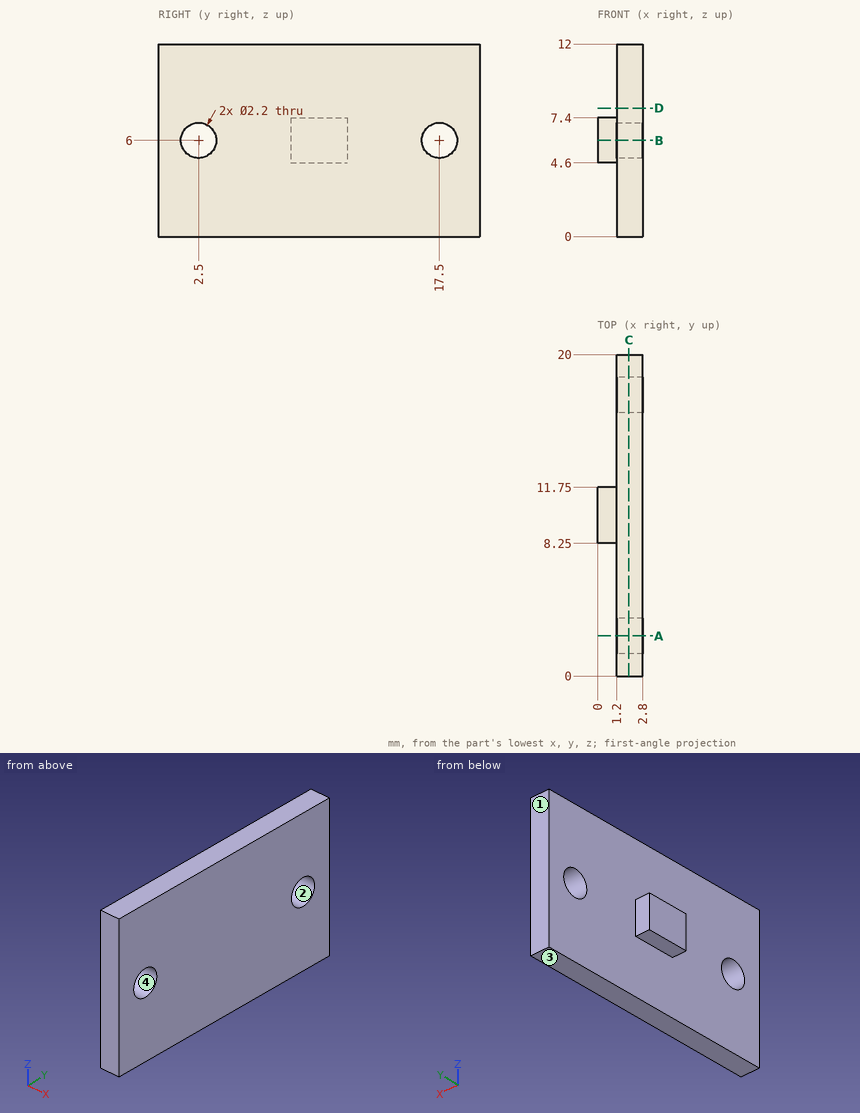
Could you check a few things on this drawing? It's one solid part, dimensions in mm from its lowest x, y, z. Coordinates: 2 decimals unless noted, no trailing zeros. Order: outer loops, then holes, each group sorted by start corner. A loop starts at its lowest first (then second) coordinate and runs counter-clockwise, first axis right, second up. Notation, with made-up numbers: M -30.5,35 L 2.5,35 A27 cw 2.5,60 Z; hole C 37.25,-19.5 d9. An arc over 180 degrees is marked long. Use one line per item in the form item = value. Start each with the question number.
1. Suppose I cut it at A-A on y = 2.5. Write out the boundary of the cut face in (x, z).
2. Suppose I cut it at C-C on x = 1.95. Write out the boundary of the cut face in (y, z), then the cut area to 3 significant figures.
3. Suppose I cut it at D-D on z = 8. Write out the boundary of the cut face in (x, y).
4. Please list where these lines run through material, in increasing order: line 1 (Y direction, x = 2.45, z = 6); line 2 (X direction, y = 6.75, z = 1.75); line 3 (Z direction, x = 2.2, y = 3.25).
5. We'd pull the mould along Z, two halves only. Please class the marked faces 1, 2, 3 and 4: +Z half, -Z half, draft (parallel to the pull), parting line (faces both ways), or undercut.
6. For pin 1 (1 mm diameter, centred on y = 5.5, z = 9.5, fed in from -X); pin 2 (1.3 mm diameter, centred on x = 0.5, z = 6.5, fed in from +Y); pin 3 (0.6 mm diameter, centred on x = 0.5, y = 10.5, fed in from +Z), each with a flat end and sliding along its axis, tell me the tip position at first contact or that it passes through.
7. Suppose I cut it at B-B on z = 6. Write out the boundary of the cut face in (x, y).
Geometry says:
q1.outline = M 1.2,0 L 2.8,0 L 2.8,4.9 L 1.2,4.9 Z; M 1.2,7.1 L 2.8,7.1 L 2.8,12 L 1.2,12 Z
q2.outline = M 0,0 L 20,0 L 20,12 L 0,12 Z; hole C 2.5,6 d2.2; hole C 17.5,6 d2.2
q2.area = 232 mm^2
q3.outline = M 1.2,0 L 2.8,0 L 2.8,20 L 1.2,20 Z
q4.line_1 = 0 to 1.4, 3.6 to 16.4, 18.6 to 20
q4.line_2 = 1.2 to 2.8
q4.line_3 = 0 to 5.2, 6.8 to 12
q5.face_1 = draft
q5.face_2 = undercut
q5.face_3 = -Z half
q5.face_4 = undercut
q6.pin_1 = 1.2
q6.pin_2 = 11.75
q6.pin_3 = 7.4
q7.outline = M 0,8.25 L 1.2,8.25 L 1.2,3.6 L 2.8,3.6 L 2.8,16.4 L 1.2,16.4 L 1.2,11.75 L 0,11.75 Z; M 1.2,0 L 2.8,0 L 2.8,1.4 L 1.2,1.4 Z; M 1.2,18.6 L 2.8,18.6 L 2.8,20 L 1.2,20 Z
